Design review of the part built by this model. Coordinates are the model's own, in mm. Face numbers are marked on the shaded views. A direction names the side the tool comes from. Round coordinates to 2 decimals unless told otherwise and drop trailing zeros. Order: outer loops, then holes, each group sorted by start corner. A loop starts at its lowest first (then second) coordinate and runs counter-clockwise, first axis right, second up. Notation, with made-up numbers: (59, -21.5) - (69, -21.5) arc R13 ccw to (69, 0.5) - close; hole circle Ø4 at (-32.75, 1). An arc over 180 degrees is marked (long way). Use CSV: the item, a comma, the result in double quotes.
from build123d import *

# Parameters (mm, degrees)
ORTHOGONAL_START                              = -15
ORTHOGONAL_CHASSIS_PLATE_PRIMARY_PROFILE_W    = 66
ORTHOGONAL_CHASSIS_PLATE_PRIMARY_PROFILE_H    = 4
ORTHOGONAL_CHASSIS_PLATE_PRIMARY_DEPTH        = 25.1
ORTHOGONAL_START_2                            = 10
ORTHOGONAL_CHASSIS_PLATE_GUIDE_SIDE_PROF_W    = 109
ORTHOGONAL_CHASSIS_PLATE_GUIDE_SIDE_PROF_H    = 4
ORTHOGONAL_CHASSIS_PLATE_GUIDE_SIDE_DEPTH     = 43
HORIZONTAL_START                              = 20
HORIZONTAL_SERVO_SEAT_UPRIGHTS_PROFILE_W      = 7.5
HORIZONTAL_SERVO_SEAT_UPRIGHTS_PROFILE_H      = 37.1
HORIZONTAL_SERVO_SEAT_UPRIGHTS_PROFILE_W_2    = 10
HORIZONTAL_SERVO_SEAT_UPRIGHTS_DEPTH          = 6
SIDE_START                                    = 27.5
SIDE_MOUNTING_FACE_FOR_MGN7_RAIL_PROFILE_W    = 100
SIDE_MOUNTING_FACE_FOR_MGN7_RAIL_PROFILE_H    = 16.6
SIDE_MOUNTING_FACE_FOR_MGN7_RAIL_DEPTH        = 4.9
HORIZONTAL_START_2                            = 49
HORIZONTAL_LIMIT_BRACKET_FOOT_SUPPORT_PR_W    = 18
HORIZONTAL_LIMIT_BRACKET_FOOT_SUPPORT_PR_H    = 5.1
HORIZONTAL_LIMIT_BRACKET_FOOT_SUPPORT_DEPTH   = 4
CHASSIS_START                                 = 28.9
CHASSIS_MOUNTING_HOLE_LAYOUT_45_X_41_2_R      = 1.6
CHASSIS_MOUNTING_HOLE_LAYOUT_45_X_41_MM_DEPTH = 4.2
SERVO_START                                   = 19.9
SERVO_MOUNT_50_X_10_MM_PITCH_PROFILE_R        = 1.6
SERVO_MOUNT_50_X_10_MM_PITCH_DEPTH            = 6.2
GUIDE_START                                   = 27.45
GUIDE_M2_MOUNTING_PILOTS_15_MM_PITCH_PRO_R    = 1.05
GUIDE_M2_MOUNTING_PILOTS_15_MM_PITCH_DEPTH    = 5.05
STOP_START                                    = 48.9
STOP_MOUNTING_TWO_M3_PILOTS_10_MM_PI_2_R      = 1.6
STOP_MOUNTING_TWO_M3_PILOTS_10_MM_PITCH_DEPTH = 4.2
FILLET_2_R                                    = 3
SKETCH_3_W                                    = 18
SKETCH_3_H                                    = 3
CUT_EXTRUDE_1_DEPTH                           = 2
CUT_EXTRUDE_2_DEPTH                           = 2.4
EXTRUDE_3_DEPTH                               = 7.5
EXTRUDE_4_DEPTH                               = 10
FILLET_3_R                                    = 5
SKETCH_7_W                                    = 109
SKETCH_7_H                                    = 1.5
CUT_EXTRUDE_3_DEPTH                           = 80
SKETCH_8_W                                    = 23
SKETCH_8_H                                    = 43
CUT_EXTRUDE_4_DEPTH                           = 30
RAISE_START                                   = 20
RAISE_SERVO_MOUNTING_TABS_BY_4_10_MM_PRO_W    = 7.5
RAISE_SERVO_MOUNTING_TABS_BY_4_10_MM_PRO_H    = 5.1
RAISE_SERVO_MOUNTING_TABS_BY_4_10_MM_PRO_W_2  = 10
RAISE_SERVO_MOUNTING_TABS_BY_4_10_MM_DEPTH    = 6
FILL_START                                    = 20
FILL_ORIGINAL_SERVO_HOLES_PROFILE_R           = 1.65
FILL_ORIGINAL_SERVO_HOLES_DEPTH               = 6
SERVO_MOUNTING_HOLES_RAISED_4_10_MM_PROF_R    = 1.6
SERVO_MOUNTING_HOLES_RAISED_4_10_MM_DEPTH     = 6.2
EXTRUDE_5_DEPTH                               = 2


with BuildPart() as part:
    # Orthogonal chassis plate primary profile → Orthogonal chassis plate primary (new body)
    with BuildSketch(Plane.XY.offset(ORTHOGONAL_START)):
        with Locations((8, 31)):
            Rectangle(ORTHOGONAL_CHASSIS_PLATE_PRIMARY_PROFILE_W, ORTHOGONAL_CHASSIS_PLATE_PRIMARY_PROFILE_H)
    extrude(amount=ORTHOGONAL_CHASSIS_PLATE_PRIMARY_DEPTH)

    # Orthogonal chassis plate guide side profile → Orthogonal chassis plate guide side (add)
    with BuildSketch(Plane.XY.offset(ORTHOGONAL_START_2)):
        with Locations((29.5, 31)):
            Rectangle(ORTHOGONAL_CHASSIS_PLATE_GUIDE_SIDE_PROF_W, ORTHOGONAL_CHASSIS_PLATE_GUIDE_SIDE_PROF_H)
    extrude(amount=ORTHOGONAL_CHASSIS_PLATE_GUIDE_SIDE_DEPTH)

    # Horizontal servo seat uprights profile → Horizontal servo seat uprights (add)
    with BuildSketch(Plane.XY.offset(HORIZONTAL_START)):
        with Locations((-14.75, 10.55)):
            Rectangle(HORIZONTAL_SERVO_SEAT_UPRIGHTS_PROFILE_W, HORIZONTAL_SERVO_SEAT_UPRIGHTS_PROFILE_H)
        with Locations((36, 10.55)):
            Rectangle(HORIZONTAL_SERVO_SEAT_UPRIGHTS_PROFILE_W_2, HORIZONTAL_SERVO_SEAT_UPRIGHTS_PROFILE_H)
    extrude(amount=HORIZONTAL_SERVO_SEAT_UPRIGHTS_DEPTH)

    # Side mounting face for MGN7 rail profile → Side mounting face for MGN7 rail (add)
    with BuildSketch(Plane.XY.offset(SIDE_START)):
        with Locations((33, 20.8)):
            Rectangle(SIDE_MOUNTING_FACE_FOR_MGN7_RAIL_PROFILE_W, SIDE_MOUNTING_FACE_FOR_MGN7_RAIL_PROFILE_H)
    extrude(amount=SIDE_MOUNTING_FACE_FOR_MGN7_RAIL_DEPTH)

    # Horizontal limit bracket foot support profile → Horizontal limit bracket foot support (add)
    with BuildSketch(Plane.XY.offset(HORIZONTAL_START_2)):
        with Locations((0, 26.55)):
            Rectangle(HORIZONTAL_LIMIT_BRACKET_FOOT_SUPPORT_PR_W, HORIZONTAL_LIMIT_BRACKET_FOOT_SUPPORT_PR_H)
    extrude(amount=HORIZONTAL_LIMIT_BRACKET_FOOT_SUPPORT_DEPTH)

    # Chassis mounting hole layout 45 x 41 2 → Chassis mounting hole layout 45 x 41 mm (cut)
    with BuildSketch(Plane(origin=(0, 0, 0), x_dir=(1, 0, 0), z_dir=(0, 1, 0)).offset(CHASSIS_START)):
        with Locations(Location((-19.5, 10.5, 0), (0, 0, 90))):
            Circle(CHASSIS_MOUNTING_HOLE_LAYOUT_45_X_41_2_R)
        with Locations(Location((-19.5, -48.5, 0), (0, 0, 90))):
            Circle(CHASSIS_MOUNTING_HOLE_LAYOUT_45_X_41_2_R)
        with Locations(Location((25.5, 10.5, 0), (0, 0, 90))):
            Circle(CHASSIS_MOUNTING_HOLE_LAYOUT_45_X_41_2_R)
        with Locations(Location((25.5, -48.5, 0), (0, 0, 90))):
            Circle(CHASSIS_MOUNTING_HOLE_LAYOUT_45_X_41_2_R)
        with Locations(Location((70.5, -48.5, 0), (0, 0, 90))):
            Circle(CHASSIS_MOUNTING_HOLE_LAYOUT_45_X_41_2_R)
    extrude(amount=CHASSIS_MOUNTING_HOLE_LAYOUT_45_X_41_MM_DEPTH, mode=Mode.SUBTRACT)

    # Servo mount 50 x 10 mm pitch profile → Servo mount 50 x 10 mm pitch (cut)
    with BuildSketch(Plane.XY.offset(SERVO_START)):
        with Locations(Location((-15, -5, 0), (0, 0, 180))):
            Circle(SERVO_MOUNT_50_X_10_MM_PITCH_PROFILE_R)
        with Locations(Location((-15, 5, 0), (0, 0, 180))):
            Circle(SERVO_MOUNT_50_X_10_MM_PITCH_PROFILE_R)
        with Locations(Location((35, -5, 0), (0, 0, 180))):
            Circle(SERVO_MOUNT_50_X_10_MM_PITCH_PROFILE_R)
        with Locations(Location((35, 5, 0), (0, 0, 180))):
            Circle(SERVO_MOUNT_50_X_10_MM_PITCH_PROFILE_R)
    extrude(amount=SERVO_MOUNT_50_X_10_MM_PITCH_DEPTH, mode=Mode.SUBTRACT)

    # Guide M2 mounting pilots 15 mm pitch profile → Guide M2 mounting pilots 15 mm pitch (cut)
    with BuildSketch(Plane.XY.offset(GUIDE_START)):
        with Locations((-12, 19)):
            Circle(GUIDE_M2_MOUNTING_PILOTS_15_MM_PITCH_PRO_R)
        with Locations((3, 19)):
            Circle(GUIDE_M2_MOUNTING_PILOTS_15_MM_PITCH_PRO_R)
        with Locations((18, 19)):
            Circle(GUIDE_M2_MOUNTING_PILOTS_15_MM_PITCH_PRO_R)
        with Locations((33, 19)):
            Circle(GUIDE_M2_MOUNTING_PILOTS_15_MM_PITCH_PRO_R)
        with Locations((48, 19)):
            Circle(GUIDE_M2_MOUNTING_PILOTS_15_MM_PITCH_PRO_R)
        with Locations((63, 19)):
            Circle(GUIDE_M2_MOUNTING_PILOTS_15_MM_PITCH_PRO_R)
        with Locations((78, 19)):
            Circle(GUIDE_M2_MOUNTING_PILOTS_15_MM_PITCH_PRO_R)
    extrude(amount=GUIDE_M2_MOUNTING_PILOTS_15_MM_PITCH_DEPTH, mode=Mode.SUBTRACT)

    # Stop mounting two M3 pilots 10 mm pi 2 → Stop mounting two M3 pilots 10 mm pitch (cut)
    with BuildSketch(Plane.XY.offset(STOP_START)):
        with Locations((-5, 27)):
            Circle(STOP_MOUNTING_TWO_M3_PILOTS_10_MM_PI_2_R)
        with Locations((5, 27)):
            Circle(STOP_MOUNTING_TWO_M3_PILOTS_10_MM_PI_2_R)
    extrude(amount=STOP_MOUNTING_TWO_M3_PILOTS_10_MM_PITCH_DEPTH, mode=Mode.SUBTRACT)

    # 圆角2
    # the kernel refuses this fillet: 3 mm, written as the material it adds along each edge
    with BuildSketch(Plane(origin=(-17, 29, 27.5), x_dir=(0, 0, -1), z_dir=(1, 0, 0))) as fillet_2_piece_1:
        with BuildLine():
            CenterArc((FILLET_2_R, -FILLET_2_R), FILLET_2_R, 90, 90)
            Line((0, -FILLET_2_R), (0, 0))
            Line((0, 0), (FILLET_2_R, 0))
        make_face()
    extrude(amount=100)

    # 草图3 → 切除-拉伸1 (cut)
    with BuildSketch(Plane(origin=(0, 29, 0), x_dir=(-1, 0, 0), z_dir=(0, -1, 0))):
        with Locations((0, -47.5)):
            Rectangle(SKETCH_3_W, SKETCH_3_H)
    extrude(amount=-CUT_EXTRUDE_1_DEPTH, mode=Mode.SUBTRACT)

    # 草图4 → 切除-拉伸2 (cut)
    with BuildSketch(Plane(origin=(0, 0, 49), x_dir=(-1, 0, 0), z_dir=(0, 0, -1))):
        Polygon((-3.267949192, 30), (-6.732050808, 30), (-8.464101615, 27), (-6.732050808, 24), (-3.267949192, 24), (-1.535898385, 27), align=None)
        Polygon((6.732050808, 30), (3.267949192, 30), (1.535898385, 27), (3.267949192, 24), (6.732050808, 24), (8.464101615, 27), align=None)
    extrude(amount=-CUT_EXTRUDE_2_DEPTH, mode=Mode.SUBTRACT)

    # 草图5 → 凸台-拉伸3 (add)
    with BuildSketch(Plane(origin=(-11, 0, 0), x_dir=(0, 0, -1), z_dir=(1, 0, 0))):
        Polygon((-20, 29), (5, 29), (-20, 9), align=None)
    extrude(amount=-EXTRUDE_3_DEPTH)

    # 草图6 → 凸台-拉伸4 (add)
    with BuildSketch(Plane.ZY.offset(-31)):
        Polygon((20, 29), (-5, 29), (20, 9), align=None)
    extrude(amount=-EXTRUDE_4_DEPTH)

    # 圆角3
    fillet_3_edges = [part.edges().sort_by_distance(p)[0] for p in [
        (-14.75, 9, 20),
        (-14.75, 29, -5),
        (36, 9, 20),
        (36, 29, -5),
    ]]
    fillet(fillet_3_edges, radius=FILLET_3_R)

    # 草图7 → 切除-拉伸3 (cut)
    with BuildSketch(Plane.XY.offset(53)):
        with Locations((29.5, 32.25)):
            Rectangle(SKETCH_7_W, SKETCH_7_H)
    extrude(amount=-CUT_EXTRUDE_3_DEPTH, mode=Mode.SUBTRACT)

    # 草图8 → 切除-拉伸4 (cut)
    with BuildSketch(Plane(origin=(0, 31.5, 0), x_dir=(1, 0, 0), z_dir=(0, 1, 0))):
        with Locations((72.5, -31.5)):
            Rectangle(SKETCH_8_W, SKETCH_8_H)
    extrude(amount=-CUT_EXTRUDE_4_DEPTH, mode=Mode.SUBTRACT)

    # Raise servo mounting tabs by 4.10 mm profile → Raise servo mounting tabs by 4.10 mm (add)
    with BuildSketch(Plane.XY.offset(RAISE_START)):
        with Locations((-14.75, -9.55)):
            Rectangle(RAISE_SERVO_MOUNTING_TABS_BY_4_10_MM_PRO_W, RAISE_SERVO_MOUNTING_TABS_BY_4_10_MM_PRO_H)
        with Locations((36, -9.55)):
            Rectangle(RAISE_SERVO_MOUNTING_TABS_BY_4_10_MM_PRO_W_2, RAISE_SERVO_MOUNTING_TABS_BY_4_10_MM_PRO_H)
    extrude(amount=RAISE_SERVO_MOUNTING_TABS_BY_4_10_MM_DEPTH)

    # Fill original servo holes profile → Fill original servo holes (add)
    with BuildSketch(Plane.XY.offset(FILL_START)):
        with Locations((-15, -5)):
            Circle(FILL_ORIGINAL_SERVO_HOLES_PROFILE_R)
        with Locations((-15, 5)):
            Circle(FILL_ORIGINAL_SERVO_HOLES_PROFILE_R)
        with Locations((35, -5)):
            Circle(FILL_ORIGINAL_SERVO_HOLES_PROFILE_R)
        with Locations((35, 5)):
            Circle(FILL_ORIGINAL_SERVO_HOLES_PROFILE_R)
    extrude(amount=FILL_ORIGINAL_SERVO_HOLES_DEPTH)

    # Servo mounting holes raised 4.10 mm profile → Servo mounting holes raised 4.10 mm (cut)
    with BuildSketch(Plane.XY.offset(SERVO_START)):
        with Locations(Location((-15, -9.1, 0), (0, 0, 180))):
            Circle(SERVO_MOUNTING_HOLES_RAISED_4_10_MM_PROF_R)
        with Locations(Location((-15, 0.9, 0), (0, 0, 180))):
            Circle(SERVO_MOUNTING_HOLES_RAISED_4_10_MM_PROF_R)
        with Locations(Location((35, -9.1, 0), (0, 0, 180))):
            Circle(SERVO_MOUNTING_HOLES_RAISED_4_10_MM_PROF_R)
        with Locations(Location((35, 0.9, 0), (0, 0, 180))):
            Circle(SERVO_MOUNTING_HOLES_RAISED_4_10_MM_PROF_R)
    extrude(amount=SERVO_MOUNTING_HOLES_RAISED_4_10_MM_DEPTH, mode=Mode.SUBTRACT)

    # 草图9 → 凸台-拉伸5 (add)
    with BuildSketch(Plane(origin=(41, 0, 0), x_dir=(0, 0, -1), z_dir=(1, 0, 0))):
        Polygon((-24.5, 29), (6.753905297, 29), (-20, -12.1), align=None)
    extrude(amount=-EXTRUDE_5_DEPTH)


solid = part.part
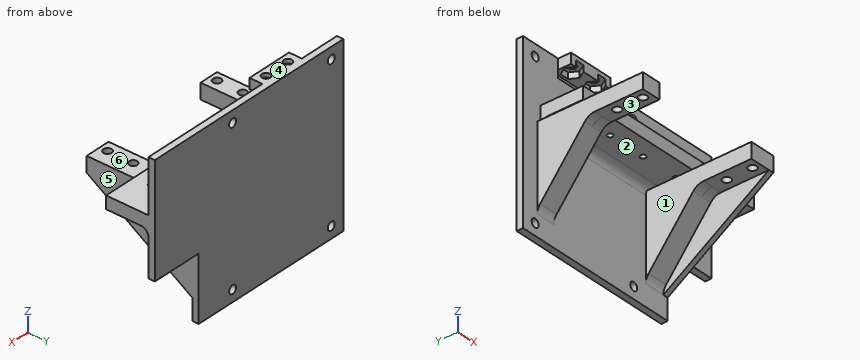
1) We need section C-C (y = 19). Give the number of separate pieces and of enclosed holes in the cut face, then the cut area to 3 significant figures.
Data:
separate pieces,"8"
enclosed holes,"0"
area,"670 mm2"
2) We need section D-D (x = 56.5). Give the boundary of the cut face in (y, z).
Data:
outline,"(12.5, 27.5) - (26, 27.5) arc R3 cw to (29, 24.5) - (29, 10) - (31.5, 10) - (31.5, 53) - (29, 53) - (29, 32.4) - (12.5, 32.4) - close"
3) Insertion check: pin 1 Ø2.5 at (x, y) = (3, 19) entering from +Z; pin 2 Ø2 at (x, z) = (33.5, -2.5) entering from -Y; pin 3 Ø4 at (x, y) = (19.5, 16) entering from -Z. Each pin has a flat end and moves straight along its axis. Give the tip position at first contact, or say it passes through.
Data:
pin 1,"stops at z = 32.4"
pin 2,"stops at y = 26.2"
pin 3,"stops at z = 27.5"
4) For the marked faces 1, 2 and 3, list the 3-axis set-ups (+Z, -Z, +X, -X, +Y, -Y) from which the entire face can be reached by the end or side of a thin tool; tool diameter is ignored.
Data:
face 1,"-Z, -Y"
face 2,"+X, -X, -Y"
face 3,"-Z, -X, -Y"
5) The part is to be moulded in two halves that separate along Z. For the marked faces 4, 5 and 6, say which applies: +Z half, -Z half, draft (parallel to the pull), parting line (faces both ways), or undercut.
Data:
face 4,"+Z half"
face 5,"draft"
face 6,"undercut"
6) We need section A-A (x = 18). Give the boundary of the cut face in (y, z), then the cut area to 3 significant figures.
Data:
outline,"(12.5, 27.5) - (17.95, 27.5) - (17.95, 32.4) - (12.5, 32.4) - close; (20.05, 27.5) - (26, 27.5) arc R3 cw to (29, 24.5) - (29, -15) - (31.5, -15) - (31.5, 53) - (29, 53) - (29, 32.4) - (20.05, 32.4) - close"
area,"242 mm2"
7) To check wall thickness, follow L1, parallel to Y at x = -15, z = 21; L2, parallel to X at y = 19, z = 30.1; L3, parallel to X at y = -6.5, z = 24. State the ranges of each line that lie inside material, in increasing order. Write a range as from..to.
Data:
L1,"y = -12.1..-10.7, -7.5..-0.7, 2.5..31.5"
L2,"x = -17..-13.05, -10.95..1.95, 4.05..16.95, 19.05..31.95, 34.05..46.95, 49.05..61"
L3,"x = -18.5..-11, 31..41"
8) We need section B-B (z = -10.5). Give the boundary of the cut face in (x, y), then the cut area to 3 significant figures.
Data:
outline,"(-25, 29) - (-21.1, 29) - (-21.1, 31.5) - (-25, 31.5) - close; (-17.9, 29) - (23.9, 29) - (23.9, 31.5) - (-17.9, 31.5) - close; (27.1, 29) - (41, 29) - (41, 31.5) - (27.1, 31.5) - close"
area,"149 mm2"
